Geometry check sheet. Reference: the model listing, model coordinates, mm. Face numbers are marked on the shaded views. A direction names the side the tool comes from. Round coordinates to 2 decimals unless told otherwise and drop trailing zeros. Loops run counter-clockwise (first coordinate to the right, second up) from the corner with the lowest first, then second, coordinate; pieces in that order, holes last. Notation, with made-up numbers: (42.25, 69.5) -> (80.25, 69.5) arc R21 ccw to (80.25, 103.5) -> close; hole circle Ø7 at (-31.5, -4.75). An arc over 180 degrees is marked (long way). Use a Markdown table: item, result. Add a question column.
Q1. Sectioned sample at A-A, the plane z = 0. Enter the section's corners in (x, y), then the cut area to 3 significant figures.
Q2. Material ranges on L1, parallel to X at y = 40, z = -13; L2, parallel to Y at x = -35, z = 17.5; L3, parallel to Z at x = -26, y = 59, recorded low to high.
Q3. Release check for a two-part mould opening along X. For the marked faces 1, 2 and 3 record: released by +X, released by -X, zero draft, split by the parting line, or undercut.
Q4. Sectioned sample at C-C, the plane y = 9. Enter the section's corners in (x, z).
Q5. Sectioned sample at B-B, the plane x = -35. Enter the section's corners in (y, z), then the cut area to 3 significant figures.
Q6. Gauge pin test, flat ends, axial feed: P1, Ø6, axis at y = 32.5, z = -13, coming from the +X side; P2, Ø6, axis at x = 39.5, z = -12, coming from the +Y side; P3, Ø1, axis at y = 11.5, z = -1.5, coming from the +X side. Record the tip position at first contact, or that the pin passes through.
Q7. Sectioned sample at D-D, the plane x = 21.5. Enter the section's corners in (y, z).
Q8. Set-up check for the marked faces 4, 5, 6 and 7: record each of +Z, -Z, +X, -X, +Y, -Y from which the full face is reachable in a straight line by a thin tool's end or side.
```python
from build123d import *

# Parameters (mm, degrees)
SKETCH2_R           = 22
BOSS_EXTRUDE1_DEPTH = 16
CUT_EXTRUDE1_DEPTH  = 17
BOSS_EXTRUDE2_DEPTH = 12
FILLET1_R           = 2


with BuildPart() as part:
    # Sketch2 → Boss-Extrude1 (new body)
    with BuildSketch(Plane(origin=(0, 0, 0), x_dir=(1, 0, 0), z_dir=(0, 1, 0))):
        with BuildLine():
            Line((37.000000064, 22), (-59, 22))
            Line((-59, 22), (-59, -22))
            Line((-59, -22), (37, -22))
            ThreePointArc((37, -22), (15, 3.2e-08), (37.000000064, 22))
        make_face()
        with Locations((37, 0)):
            Circle(SKETCH2_R)
    extrude(amount=BOSS_EXTRUDE1_DEPTH)

    # Sketch5 → Cut-Extrude1 (cut, through all)
    with BuildSketch(Plane(origin=(0, 16, 0), x_dir=(1, 0, 0), z_dir=(0, 1, 0))):
        with BuildLine():
            Line((37, -8), (12, -8))
            ThreePointArc((12, -8), (4, 0), (12, 8))
            Line((12, 8), (37, 8))
            ThreePointArc((37, 8), (45, 0), (37, -8))
        make_face()
    extrude(amount=-CUT_EXTRUDE1_DEPTH, mode=Mode.SUBTRACT)

    # Sketch6 → Boss-Extrude2 (add)
    with BuildSketch(Plane.XY.offset(22)):
        with BuildLine():
            ThreePointArc((-59, 40), (-51.970562748, 23.029437252), (-35, 16))
            ThreePointArc((-35, 16), (-18.029437252, 23.029437252), (-11, 40))
            Line((-11, 40), (-25, 40))
            ThreePointArc((-25, 40), (-35, 30), (-45, 40))
            Line((-45, 40), (-59, 40))
        make_face()
        with BuildLine():
            ThreePointArc((-11, 40), (-35, 64), (-59, 40))
            Line((-59, 40), (-45, 40))
            ThreePointArc((-45, 40), (-35, 50), (-25, 40))
            Line((-25, 40), (-11, 40))
        make_face()
        with BuildLine():
            ThreePointArc((-11, 40), (-18.029437252, 23.029437252), (-35, 16))
            Line((-35, 16), (-11, 16))
            Line((-11, 16), (-11, 40))
        make_face()
        with BuildLine():
            Line((-59, 40), (-59, 16))
            Line((-59, 16), (-35, 16))
            ThreePointArc((-35, 16), (-51.970562748, 23.029437252), (-59, 40))
        make_face()
    boss_extrude2 = extrude(amount=-BOSS_EXTRUDE2_DEPTH)

    # Mirror1: Boss-Extrude2 across plane
    add(boss_extrude2.mirror(Plane.XY))

    # Fillet1
    fillet1_edges = [part.edges().sort_by_distance(p)[0] for p in [
        (-11, 16, 16),
        (-35, 16, 10),
        (-35, 16, -10),
        (-11, 16, -16),
    ]]
    fillet(fillet1_edges, radius=FILLET1_R)


solid = part.part
```
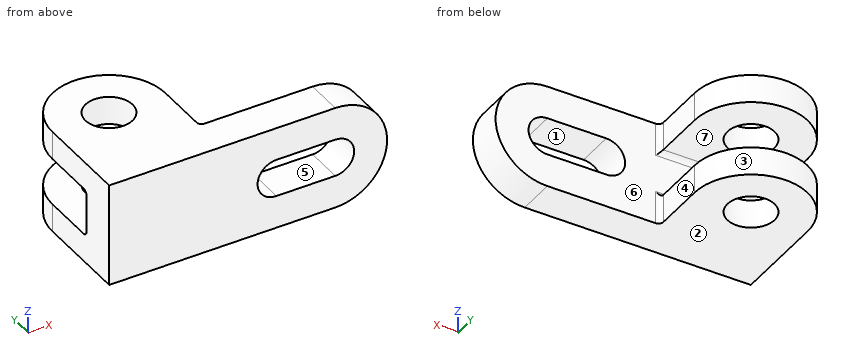
Values:
| question | item | result |
|---|---|---|
| 1 | outline | (-59, 0) -> (4, 0) -> (4, 16) -> (-59, 16) -> close; (45, 0) -> (59, 0) -> (59, 16) -> (45, 16) -> close |
| 1 | area | 1,230 mm^2 |
| 2 | L1 | -59 to -45, -25 to -11 |
| 2 | L2 | 0 to 30, 50 to 64 |
| 2 | L3 | -22 to -10, 10 to 22 |
| 3 | face 1 | undercut |
| 3 | face 2 | zero draft |
| 3 | face 3 | split by the parting line |
| 4 | outline | (-59, -22) -> (37, -22) arc R22 ccw to (37, 22) -> (-59, 22) -> close; hole (12, -8) -> (37, -8) arc R8 ccw to (37, 8) -> (12, 8) arc R8 ccw to start |
| 5 | outline | (0, -22) -> (30, -22) -> (30, -10) -> (18, -10) arc R2 cw to (16, -8) -> (16, 8) arc R2 cw to (18, 10) -> (30, 10) -> (30, 22) -> (0, 22) -> close; (50, -22) -> (64, -22) -> (64, -10) -> (50, -10) -> close; (50, 10) -> (64, 10) -> (64, 22) -> (50, 22) -> close |
| 5 | area | 1,380 mm^2 |
| 6 | P1 | x = -11 |
| 6 | P2 | y = 16 |
| 6 | P3 | x = 58.98 |
| 7 | outline | (0, -22) -> (16, -22) -> (16, -8) -> (0, -8) -> close; (0, 8) -> (16, 8) -> (16, 22) -> (0, 22) -> close |
| 8 | face 4 | +Z, -Z, +X, +Y |
| 8 | face 5 | +Y, -Y |
| 8 | face 6 | +X, +Y |
| 8 | face 7 | +X, -X, +Y |
